Source: CAD feature listing. Evaluate the final solid. Frame: model axes, mm. Face numbers are marked on the shaded views. Round coordinates to 2 decimals unless told otherwise and drop trailing zeros. Loops run counter-clockwise (first coordinate to the right, second up) from the corner with the lowest first, then second, coordinate; pieces in that order, holes last. Notation, with made-up numbers: (-9, 49.25) -> (2, 49.25) arc R14 cw to (2, 68.25) -> close; hole circle Ø4 at (-15.75, 48). An arc over 180 degrees is marked (long way). Put each result on its own line as item: value. Start each with the question number.
1. Cut plane D-D (z = 1.4). Return the cut outline in (x, y), then the cut area to 3 significant figures.
2. Cut plane A-A (y = -1.5). Return the cut outline in (x, z), then the cut area to 3 significant figures.
3. Cut plane B-B (x = 5.25). Return the cut outline in (y, z).
4. Material intervals for L1, parallel to X at y = -0.5, z = 1.3; L2, parallel to Y at x = 4.75, z = 1.5; L3, parallel to Y at x = 0.75, z = 0.95, sorted ascending.
5. Cut plane C-C (z = 0.75). Return the cut outline in (x, y).
6. Contact query for flat-ended pins moving along their axis: pin 1 (0.5 mm diameter, centred on x = 1, y = -2.5, fed in from +Z); pin 2 (0.7 mm diameter, centred on x = 1, y = -0.5, fed in from -Z); pin 3 (0.5 mm diameter, centred on y = -1.5, z = 0.5, fed in from +X). Output: stop coordinate, or through.
7. Draft query along Z for the marked faces 1, 2 and 3. Return one class per face: pulls with the +Z half, pulls with the -Z half, needs draft (parallel to the pull), parting line crosses it, or undercut.
```python
from build123d import *

# Parameters (mm, degrees)
EXTRUSION1_DEPTH        = 2.2
ENL_V_MAT_EXTRU_1_DEPTH = 9.576619381


with BuildPart() as part:
    # Esquisse1 → Extrusion1 (new body)
    with BuildSketch(Plane.XY):
        Polygon((0, 0), (0.68, 0), (0.68, -3), (1.32, -3), (1.32, 0), (5.08, 0), (5.08, -3), (5.72, -3), (5.72, 0), (6.4, 0), (6.4, 6), (0, 6), align=None)
    extrude(amount=EXTRUSION1_DEPTH)

    # Esquisse2 → Enlèv. mat.-Extru.1 (cut, through all)
    with BuildSketch(Plane.ZY.offset(-0.68)):
        Polygon((0.45, -1.971195231), (0.45, -3.327188137), (4.113583834, -3.327188137), (4.113583834, 0), (1.55, 0), (1.55, -1.220350349), align=None)
        Polygon((0, -1.733519979), (0, -3.327188137), (-1.233682365, -3.327188137), (-1.233682365, 0), (1.1, 0), (1.1, -0.982675097), align=None)
    extrude(amount=-ENL_V_MAT_EXTRU_1_DEPTH, mode=Mode.SUBTRACT)


solid = part.part
```
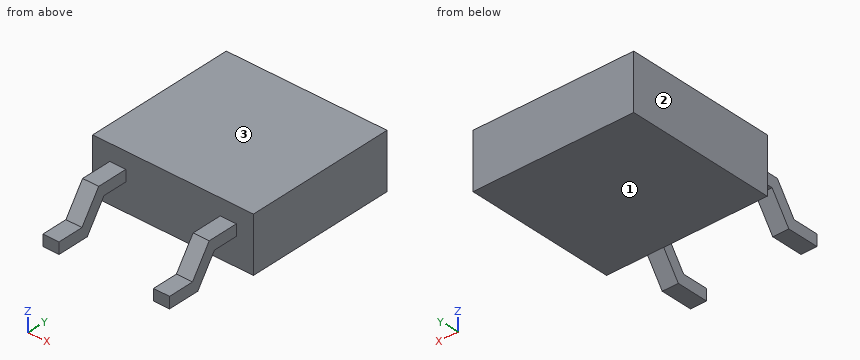
Solution:
1. outline: (0, 0) -> (0.68, 0) -> (0.68, -1.32) -> (1.32, -1.32) -> (1.32, 0) -> (5.08, 0) -> (5.08, -1.32) -> (5.72, -1.32) -> (5.72, 0) -> (6.4, 0) -> (6.4, 6) -> (0, 6) -> close
1. area: 40.1 mm^2
2. outline: (0.68, 0.34) -> (1.32, 0.34) -> (1.32, 1.14) -> (0.68, 1.14) -> close; (5.08, 0.34) -> (5.72, 0.34) -> (5.72, 1.14) -> (5.08, 1.14) -> close
2. area: 1.02 mm^2
3. outline: (-3, 0) -> (-1.73, 0) -> (-0.98, 1.1) -> (0, 1.1) -> (0, 0) -> (6, 0) -> (6, 2.2) -> (0, 2.2) -> (0, 1.55) -> (-1.22, 1.55) -> (-1.97, 0.45) -> (-3, 0.45) -> close
4. L1: x = 0.68 to 1.32, 5.08 to 5.72
4. L2: y = 0 to 6
4. L3: y = -1.63 to -1.09, 0 to 6
5. outline: (0, 0) -> (6.4, 0) -> (6.4, 6) -> (0, 6) -> close; (0.68, -1.77) -> (1.32, -1.77) -> (1.32, -1.22) -> (0.68, -1.22) -> close; (5.08, -1.77) -> (5.72, -1.77) -> (5.72, -1.22) -> (5.08, -1.22) -> close
6. pin 1: stops at z = 0.45
6. pin 2: stops at z = 1.1
6. pin 3: stops at x = 5.72
7. face 1: pulls with the -Z half
7. face 2: needs draft
7. face 3: pulls with the +Z half
